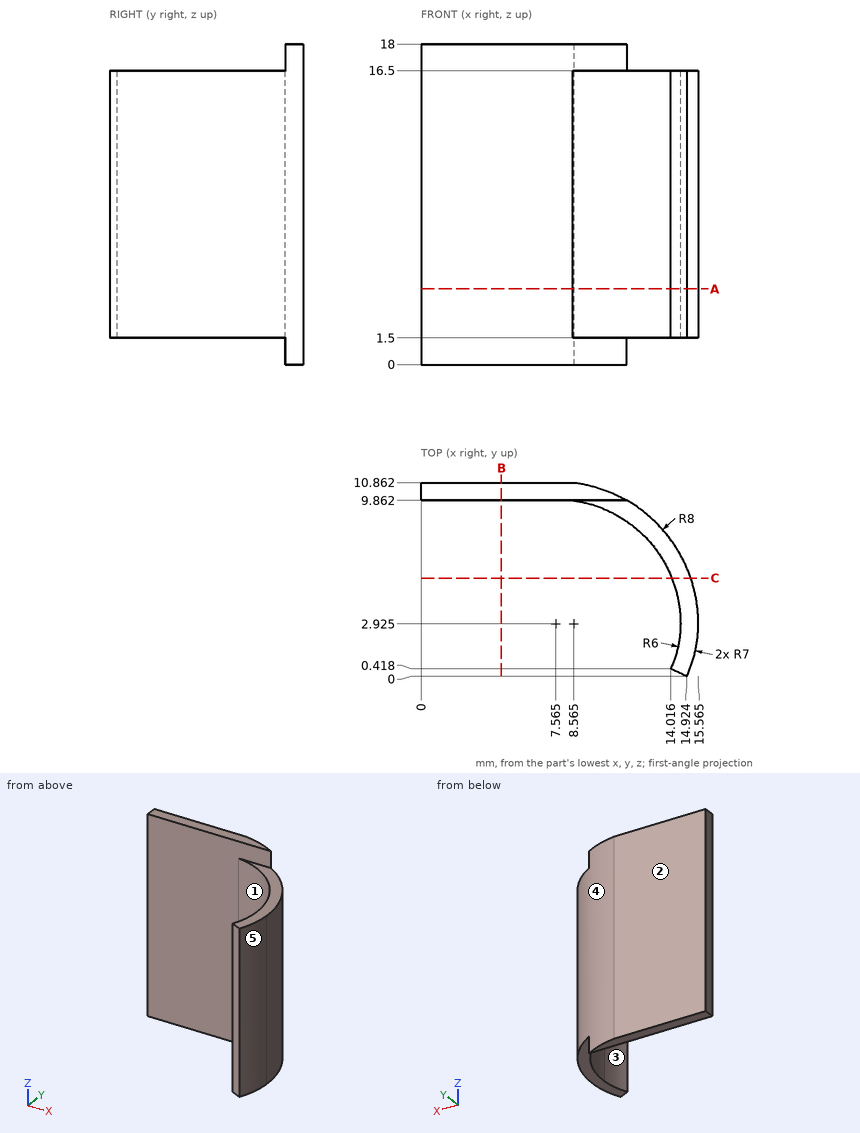
Drawing for the job (mm, zero at the part's lowest x, y, z). A direction names the side the tool comes from. Give positions to 0.01 mm unless a question says otherwise; leave off trailing zeros. Order: outer loops, then holes, each group sorted by start corner. A loop starts at its lowest first (then second) coordinate and runs counter-clockwise, first axis right, second up. Notation, with made-up numbers: M -23.5,-6.5 L 24.5,-6.5 A32 ccw 24.5,25.5 Z; hole C 53.5,7 d8. An arc over 180 degrees is marked long. Put each result on its own line as item: value.
Item 1: Slice it at B-B, the plane x = 4.5. Write the cut outline in (y, z), plus the area to 3 significant figures.
From the geometry:
outline: M 9.86,0 L 10.86,0 L 10.86,18 L 9.86,18 Z
area: 18.0 mm2
Item 2: Two-plate mould, pull along Y, no slides. Class the marked faces 3, 4 and 5: +Y half, -Y half, draft (parallel to the pull), parting line (faces both ways), or undercut.
From the geometry:
face 3: undercut
face 4: +Y half
face 5: -Y half
Item 3: Slice it at C-C, the plane y = 5.5. Write the cut outline in (x, z).
From the geometry:
outline: M 14.07,1.5 L 15.14,1.5 L 15.14,16.5 L 14.07,16.5 Z
Item 4: Flat gauge pins, fed straight in: pin 1 Ø5 at (x, z) = (5, 5) entering from -Y; pin 2 Ø2 at (y, z) = (6.5, 6) entering from -X; pin 3 Ø2 at (x, z) = (8.5, 12.5) entering from -Y; pin 4 Ø5.5 at (x, y) = (11, 3) entering from -Z. Where does each tip first touch, or does it go through?
From the geometry:
pin 1: stops at y = 9.86
pin 2: stops at x = 12.86
pin 3: stops at y = 9.65
pin 4: passes through
Item 5: Probe line 1 (Y direction, x = 3.5, z = 11); line 2 (Y direction, x = 13, z = 12) (1 decimal); line 3 (X direction, y = 5.5, z = 6) (1 decimal). List the from-to ranges inside material, lowest first. Write a range as [from, to].
From the geometry:
line 1: y = [9.86, 10.86]
line 2: y = [7.3, 8.8]
line 3: x = [14.1, 15.1]
Item 6: Slice it at A-A, the plane z = 4.25. Write the cut outline in (x, y) (1 decimal).
From the geometry:
outline: M 0,9.9 L 8.5,9.9 A7 cw 14.6,2.9 A6 cw 14,0.4 L 14.9,0 A7 ccw 15.6,2.9 A8 ccw 8.6,10.9 L 0,10.9 Z
Item 7: 3-axis set-ups, long thin cutter, end or side, ignore diameter. For the marked faces 1 and 2: which of +Z, -Z, +X, -X, +Y, -Y reach the whole face in a straight line?
From the geometry:
face 1: +Z, -Z, -X
face 2: +Z, -Z, +X, -X, +Y
